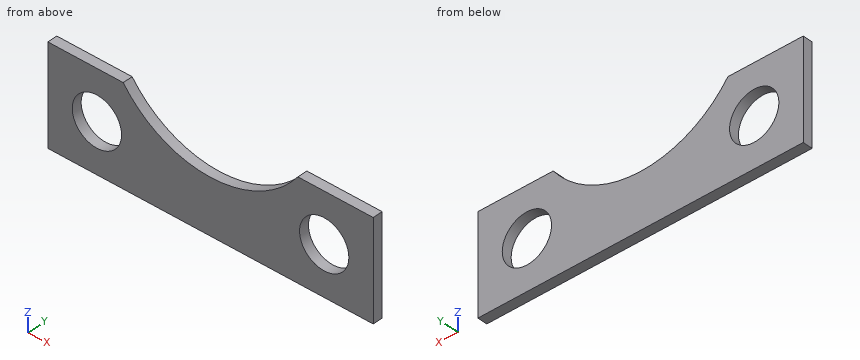
from build123d import *

# Parameters (mm, degrees)
SKETCH1_R           = 2.5
BOSS_EXTRUDE1_DEPTH = 1


with BuildPart() as part:
    # Sketch1 → Boss-Extrude1 (new body)
    with BuildSketch(Plane(origin=(0, 0, 0), x_dir=(1, 0, 0), z_dir=(0, 1, 0))):
        with BuildLine():
            Line((-16.5, 10), (16.5, 10))
            Line((16.5, 10), (16.5, 0))
            Line((16.5, 0), (8.855753779, 0))
            ThreePointArc((8.855753779, 0), (0, 4.475), (-8.855753779, 0))
            Line((-8.855753779, 0), (-16.5, 0))
            Line((-16.5, 0), (-16.5, 10))
        make_face()
        with Locations((-11.525, 5)):
            Circle(SKETCH1_R, mode=Mode.SUBTRACT)
        with Locations((11.525, 5)):
            Circle(SKETCH1_R, mode=Mode.SUBTRACT)
    extrude(amount=BOSS_EXTRUDE1_DEPTH)


solid = part.part
Read the model definition and answer for the solid it produces. Units are mm, in the model's axes. Round coordinates to 2 decimals unless told otherwise and drop trailing zeros. Order: outer loops, then holes, each group sorted by start corner. A loop starts at its lowest first (then second) coordinate and runs counter-clockwise, first axis right, second up. Notation, with made-up numbers: (65.5, 38.25) - (101.5, 38.25) arc R18 ccw to (101.5, 53.25) - close; hole circle Ø7 at (82.25, -24). An arc over 180 degrees is marked (long way). Use one line per item in the form item = value. Start each with the question number.
(1) The part is cut by section C-C (z = -3). Give the vertices of the cut face in (x, y) (3 decimals).
(2) The part is cut by section A-A (z = -5). Give the vertices of the cut face in (x, y) (3 decimals).
(3) The part is cut by section B-B (y = 0.45). Give the vertices of the cut face in (x, z) (3 decimals).
(4) Find the intervals of material crossed by line 1 along X through (y, z) = (0.7, -5) (3 decimals); line 2 along X through (y, z) = (0.4, -6.75); line 3 along Z through (x, y) = (-10, 0.35), in increasing order. Write a range as from..to.
(5) The part is cut by section D-D (x = 0). Give the vertices of the cut face in (y, z) (3 decimals).
Checked values:
q1.outline = (-16.5, 0) - (-13.025, 0) - (-13.025, 1) - (-16.5, 1) - close; (-10.025, 0) - (-5.502, 0) - (-5.502, 1) - (-10.025, 1) - close; (5.502, 0) - (10.025, 0) - (10.025, 1) - (5.502, 1) - close; (13.025, 0) - (16.5, 0) - (16.5, 1) - (13.025, 1) - close
q2.outline = (-16.5, 0) - (-14.025, 0) - (-14.025, 1) - (-16.5, 1) - close; (-9.025, 0) - (9.025, 0) - (9.025, 1) - (-9.025, 1) - close; (14.025, 0) - (16.5, 0) - (16.5, 1) - (14.025, 1) - close
q3.outline = (-16.5, -10) - (16.5, -10) - (16.5, 0) - (8.856, 0) arc R11 cw to (-8.856, 0) - (-16.5, 0) - close; hole circle Ø5 at (-11.525, -5); hole circle Ø5 at (11.525, -5)
q4.line_1 = -16.5..-14.025, -9.025..9.025, 14.025..16.5
q4.line_2 = -16.5..-13.31, -9.74..9.74, 13.31..16.5
q4.line_3 = -10..-6.98, -3.02..0
q5.outline = (0, -10) - (1, -10) - (1, -4.475) - (0, -4.475) - close
